Could you check a few things on this drawing? It's one solid part, dimensions in mm from its lowest x, y, z. A direction names the side the tool comes from. Round coordinates to 2 decimals unless told otherwise and drop trailing zeros. Write each loop counter-clockwise with the first axis right and the second up, starting at its lowest first coordinate (ties: lowest second). Pieces come first, ordered by that corner, then holes. Notation, with made-up numbers: (4.25, 89.25) -> (41.25, 89.25) arc R26 ccw to (41.25, 105.25) -> close; hole circle Ø7 at (64.25, -26.5). An arc over 180 degrees is marked (long way). Put each result on its own line as item: value. Start each with the question number.
1) Will these pins go through, and if not, where does the flat tip stop? P1, Ø1, axis at x = 4, z = 1, coming from the -Y side; P2, Ø4, axis at y = 6, z = 1, coming from the +X side.
2) We'd pull the mould along Y, two halves only. Please class the marked faces 3, 4, 5 and 6: released by +Y, released by -Y, zero draft, split by the parting line, or undercut.
3) I want a section at C-C, the plane z = 4. List the corners of the cut face in (x, y) for me, then the cut area to 3 significant figures.
4) Which directions (+Z, -Z, +X, -X, +Y, -Y) give clear straight access to the entire face, cutting with the end or side of a thin tool? Please do the marked faces 1 and 2.
5) If I drill on line 1 along Y through (x, z) = (12, 2.5); line 2 along Y through (x, z) = (18.25, 5); line 3 along Y through (x, z) = (13.25, 5.5), over which ranges is the centre line in solid material (lowest first)? Write a range as [from, to].
6) I want a section at A-A, the plane y = 12. Give the number of separate pieces and of enclosed holes in the cut face, then the cut area to 3 significant figures.
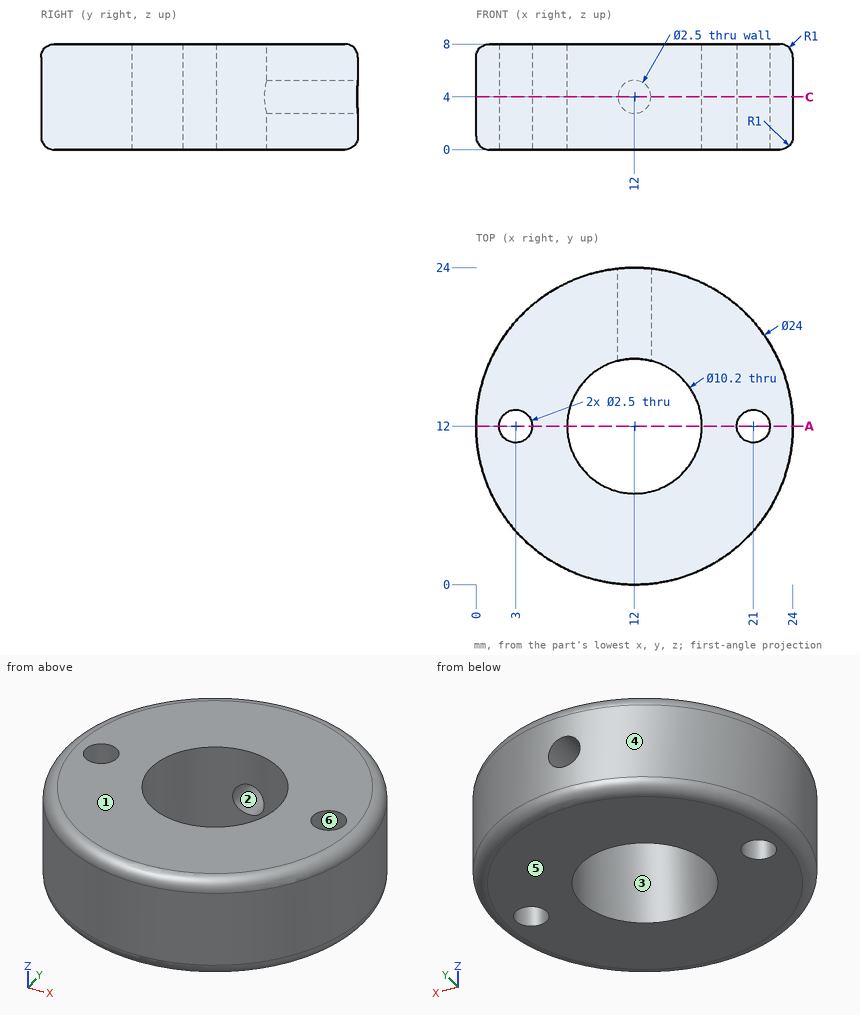
Findings:
1. P1: stops at y = 2.63
1. P2: stops at x = 23.31
2. face 3: undercut
2. face 4: split by the parting line
2. face 5: zero draft
2. face 6: undercut
3. outline: (10.75, 16.94) -> (10.75, 23.93) arc R12 ccw (long way) to (13.25, 23.93) -> (13.25, 16.94) arc R5.1 cw (long way) to start; hole circle Ø2.5 at (3, 12); hole circle Ø2.5 at (21, 12)
3. area: 344 mm2
4. face 1: +Z, +X, -X, +Y, -Y
4. face 2: +Y
5. line 1: y = [0, 6.9], [17.1, 24]
5. line 2: y = [1.76, 22.24]
5. line 3: y = [0.07, 7.06], [16.94, 23.93]
6. separate pieces: 4
6. enclosed holes: 0
6. area: 69.5 mm2
